```python
from build123d import *

# Parameters (mm, degrees)
EXTRUDE_1_DEPTH     = 5
SKETCH_2_R          = 1.25
CUT_EXTRUDE_1_DEPTH = 5


with BuildPart() as part:
    # Эскиз1 → Бобышка-Вытянуть1 (new body)
    with BuildSketch(Plane(origin=(0, 0, 0), x_dir=(1, 0, 0), z_dir=(0, 1, 0))):
        with BuildLine():
            Line((2, 0), (5, 0))
            ThreePointArc((5, 0), (3.535533906, 3.535533906), (0, 5))
            Line((0, 5), (-7, 5))
            Line((-7, 5), (-7, 0))
            Line((-7, 0), (-2, 0))
            ThreePointArc((-2, 0), (0, 2), (2, 0))
        make_face()
    extrude(amount=EXTRUDE_1_DEPTH)

    # Эскиз2 → Вырез-Вытянуть1 (cut)
    with BuildSketch(Plane.XY):
        with Locations((-4.5, 2.5)):
            Circle(SKETCH_2_R)
    extrude(amount=-CUT_EXTRUDE_1_DEPTH, mode=Mode.SUBTRACT)


solid = part.part
```
The model under review builds one solid part; all positions refer to its coordinate system, in mm. Give positions to 0.01 mm unless a question says otherwise; leave off trailing zeros. Write each loop counter-clockwise with the first axis right and the second up, starting at its lowest first coordinate (ties: lowest second). Pieces come first, ordered by that corner, then holes. Notation, with made-up numbers: (27, -32) -> (48, -32) arc R31 cw to (48, 0) -> close; hole circle Ø10 at (50, 64.5). An arc over 180 degrees is marked (long way). Answer in a Markdown table with one row per item.
1) Clearance check with a flat-ended pin moving along its axis: P1, Ø1.5, axis at x = -3, y = 4, coming from the +Z side. State where the tip first meets the part, or that it passes through.
Worked answers:
| item | result |
|---|---|
| P1 | z = 0 |
2) Add section C-C on y = 4.4. State the section outline as (x, z) points.
Worked answers:
| item | result |
|---|---|
| outline | (-7, -5) -> (0, -5) arc R5 ccw to (5, 0) -> (2, 0) arc R2 cw to (-2, 0) -> (-7, 0) -> close |
3) Add section A-A on z = -0.6. State the section outline as (x, y) points.
Worked answers:
| item | result |
|---|---|
| outline | (-7, 0) -> (-1.91, 0) -> (-1.91, 5) -> (-7, 5) -> close; (1.91, 0) -> (4.96, 0) -> (4.96, 5) -> (1.91, 5) -> close; hole circle Ø2.5 at (-4.5, 2.5) |
4) Mouldability with a two-part tool opening along Y and no side actions: class faces 1 (the flat face through (-1, 5, -3)), 2 (the cylindrical face through (-5.421, 3.345, -2.465)), 3 (the flat face through (3, 2, 0)), 4 (the flat face through (-1, 0, -3)) as +Y half, -Y half, draft (parallel to the pull), parting line (faces both ways), or undercut.
Worked answers:
| item | result |
|---|---|
| face 1 | +Y half |
| face 2 | undercut |
| face 3 | draft |
| face 4 | -Y half |
5) Add section D-D on z = -1.2. State the section outline as (x, y) points.
Worked answers:
| item | result |
|---|---|
| outline | (-7, 0) -> (-1.6, 0) -> (-1.6, 5) -> (-7, 5) -> close; (1.6, 0) -> (4.85, 0) -> (4.85, 5) -> (1.6, 5) -> close; hole circle Ø2.5 at (-4.5, 2.5) |
6) For L1, parallel to Y at x = -4.5, z = -1.15; L2, parallel to X at y = 2.95, z = -2.55; L3, parallel to Y at x = -5.25, z = -3.2, list the stretches that pass through material, from the lowest coordinate up. Write a range as [from, to].
Worked answers:
| item | result |
|---|---|
| L1 | [0, 1.25], [3.75, 5] |
| L2 | [-7, -5.67], [-3.33, 4.3] |
| L3 | [0, 1.5], [3.5, 5] |
7) Add section B-B on y = 2.85. State the section outline as (x, z) points.
Worked answers:
| item | result |
|---|---|
| outline | (-7, -5) -> (-5.7, -5) -> (-5.7, 0) -> (-7, 0) -> close; (-3.3, -5) -> (0, -5) arc R5 ccw to (5, 0) -> (2, 0) arc R2 cw to (-2, 0) -> (-3.3, 0) -> close |
